from build123d import *

# Parameters (mm, degrees)
F0_R          = 31.496
F0_R_2        = 28.956
F1_DEPTH      = 25.4
F1_DEPTH_BACK = 12.7
F3_DEPTH      = 34.925
F3_DEPTH_BACK = 34.925
F4_DEPTH      = 25.4


with BuildPart() as f1:
    # F0 (on Top) → F1 (new body, two sides)
    with BuildSketch(Plane.XY) as f1_sk:
        Circle(F0_R)
        Circle(F0_R_2, mode=Mode.SUBTRACT)
    extrude(amount=-F1_DEPTH)
    extrude(f1_sk.sketch, amount=F1_DEPTH_BACK)

    # F2 (on Right) → F3 (join, two sides)
    with BuildSketch(Plane.YZ) as f3_sk:
        with BuildLine():
            ThreePointArc((-38.9788635032, 12.7), (-20.4978157373, 3.2550660049), (0, 0))
            ThreePointArc((0, 0), (20.4978157373, 3.2550660049), (38.9788635032, 12.7))
            Line((38.9788635032, 12.7), (-38.9788635032, 12.7))
        make_face()
    extrude(amount=F3_DEPTH)
    extrude(f3_sk.sketch, amount=-F3_DEPTH_BACK)

    # F0 (on Top) → F4 (cut)
    with BuildSketch(Plane.XY):
        Circle(F0_R_2)
    extrude(amount=F4_DEPTH, mode=Mode.SUBTRACT)


solid = f1.part
Here's how the part is built. I have some questions about the finished solid (model axes, mm). A direction names the side the tool comes from. Round coordinates to 2 decimals unless told otherwise and drop trailing zeros. Order: outer loops, then holes, each group sorted by start corner. A loop starts at its lowest first (then second) coordinate and runs counter-clockwise, first axis right, second up. Notation, with made-up numbers: (59, 55.5) -> (78, 55.5) arc R13 cw to (78, 60.5) -> close; hole circle Ø6 at (19, 59.25). An arc over 180 degrees is marked (long way). Use CSV: the item, a comma, the result in double quotes.
1. I want a section at D-D on x = -23.5. List the corners of the cut face in (y, z) for me, and give its area (3 significant figures).
Recorded:
outline,"(-38.98, 12.7) arc R66.17 ccw to (-20.97, 3.41) -> (-20.97, -25.4) -> (-16.92, -25.4) -> (-16.92, 12.7) -> close; (16.92, -25.4) -> (20.97, -25.4) -> (20.97, 3.41) arc R66.17 ccw to (38.98, 12.7) -> (16.92, 12.7) -> close"
area,"497 mm2"
2. I want a section at B-B on y = 0. List the corners of the cut face in (x, z) for me (3 decimals).
Recorded:
outline,"(-34.925, 0) -> (-31.496, 0) -> (-31.496, -25.4) -> (-28.956, -25.4) -> (-28.956, 12.7) -> (-34.925, 12.7) -> close; (28.956, -25.4) -> (31.496, -25.4) -> (31.496, 0) -> (34.925, 0) -> (34.925, 12.7) -> (28.956, 12.7) -> close"
3. Which directions (+Z, -Z, +X, -X, +Y, -Y) give clear straight access to the entire face, cutting with the end or side of a thin tool? Please do faces 1 (the face through (24, 18, 12.7)), 2 (the face through (16.01, -27.51, 5.99)).
Recorded:
face 1,"+Z, +X, -X, +Y, -Y"
face 2,"-Z"
4. I'm going to push flat-ended pins straight in: P1, Ø8, axis at x = 13, z = -16.5, coming from the +Y side; P2, Ø10, axis at y = 25, z = -15, coming from the -X side; P3, Ø10, axis at y = 19, z = -17, coming from the +X side. Where does each tip first touch, or does it pass through?
Recorded:
P1,"stops at y = 30.18"
P2,"stops at x = -24.33"
P3,"stops at x = 28.21"
5. I want a section at A-A on x = 0. List the corners of the cut face in (y, z) for me.
Recorded:
outline,"(-38.98, 12.7) arc R66.17 ccw to (-31.5, 7.98) -> (-31.5, -25.4) -> (-28.96, -25.4) -> (-28.96, 12.7) -> close; (28.96, -25.4) -> (31.5, -25.4) -> (31.5, 7.98) arc R66.17 ccw to (38.98, 12.7) -> (28.96, 12.7) -> close"
6. I need wall thicknesses on line 1 along Y through (x, z) = (0, -9); line 2 along X through (y, z) = (0, 5) (3 decimals); line 3 along X through (y, z) = (-6, 9.5) (3 decimals). Which ranges of each line are inside material? Lowest first, please.
Recorded:
line 1,"y = -31.5 to -28.96, 28.96 to 31.5"
line 2,"x = -34.925 to -28.956, 28.956 to 34.925"
line 3,"x = -34.925 to -28.328, 28.328 to 34.925"
7. I want a section at C-C on z = -10.5. List the corners of the cut face in (x, y) for me.
Recorded:
outline,"circle Ø62.99 at (0, 0); hole circle Ø57.91 at (0, 0)"
